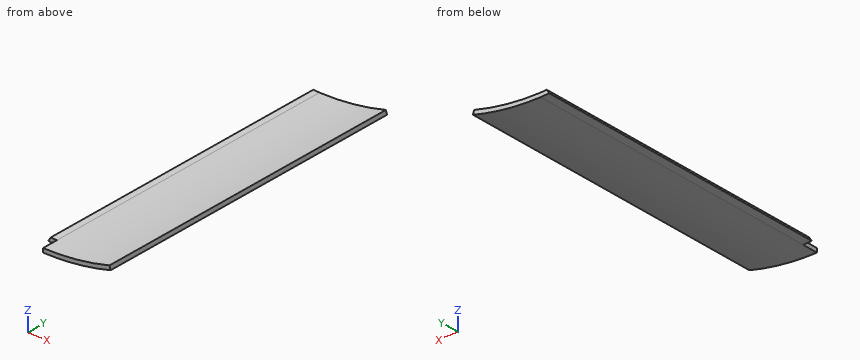
```python
from build123d import *

# Parameters (mm, degrees)
EXTRUDE_1_DEPTH = 2000
EXTRUDE_2_DEPTH = 1900


with BuildPart() as part:
    # 草图1 → 凸台-拉伸1 (new body)
    with BuildSketch(Plane(origin=(0, 0, 0), x_dir=(1, 0, 0), z_dir=(0, 1, 0))):
        with BuildLine():
            Line((0, 1540), (0, 1515))
            ThreePointArc((0, 1515), (210.847247954, 1500.256124143), (417.590594063, 1456.311469347))
            Line((417.590594063, 1456.311469347), (424.481527958, 1480.343011745))
            ThreePointArc((424.481527958, 1480.343011745), (214.326575478, 1525.012825862), (0, 1540))
        make_face()
    extrude(amount=EXTRUDE_1_DEPTH)

    # 草图2 → 凸台-拉伸2 (add)
    with BuildSketch(Plane(origin=(0, 2000, 0), x_dir=(1, 0, 0), z_dir=(0, 1, 0))):
        Polygon((-38.424352084, 1513.658192058), (0, 1515), (0, 1540), (-53.712484783, 1538.1243187), align=None)
    extrude(amount=-EXTRUDE_2_DEPTH)


solid = part.part
```
Source: CAD feature listing. Evaluate the final solid. Frame: model axes, mm. Round coordinates to 2 decimals unless told otherwise and drop trailing zeros. Order: outer loops, then holes, each group sorted by start corner. A loop starts at its lowest first (then second) coordinate and runs counter-clockwise, first axis right, second up. Notation, with made-up numbers: (-16.5, -17) -> (24.5, -17) arc R16 ccw to (24.5, 12) -> close; hole circle Ø2 at (42, 24). An arc over 180 degrees is marked (long way). One line per item, written item: value. Start each with the question number.
Q1. Pin query (flat end, axial travel): pin 1 (4 mm diameter, centred on x = 208.5, y = 636, fed in from -Z); pin 2 (7.5 mm diameter, centred on y = 60, z = -1531, fed in from -X); pin 3 (4 mm diameter, centred on y = 1010.5, z = -1527, fed in from -X). Return the tip coordinate at first contact, or that it passes through.
Q2. Section query C-C (x = 166.5). Return the cut outline in (y, z).
Q3. Section query A-A (y = 1442.5). Return the cut outline in (x, z), plus the area to 3 significant figures.
Q4. Material intervals for probe 1 along Z at (x, y) = (26, 1059.5); probe 2 along Z at (x, y) = (-7.5, 195.5), sorted ascending.
Q5. Section query B-B (x = 71). Return the cut outline in (y, z), plus the area to 3 significant figures.
Findings below:
1. pin 1: z = -1526.09
1. pin 2: x = 0
1. pin 3: x = -48.01
2. outline: (0, -1530.97) -> (2000, -1530.97) -> (2000, -1505.82) -> (0, -1505.82) -> close
3. outline: (-53.71, -1538.12) -> (0, -1540) arc R1540 ccw to (424.48, -1480.34) -> (417.59, -1456.31) arc R1515 cw to (0, -1515) -> (-38.42, -1513.66) -> close
3. area: 11,800 mm²
4. probe 1: -1539.78 to -1514.78
4. probe 2: -1539.74 to -1514.74
5. outline: (0, -1538.36) -> (2000, -1538.36) -> (2000, -1513.34) -> (0, -1513.34) -> close
5. area: 50,100 mm²
